from build123d import *

# Parameters (mm, degrees)
ESQUISSE1_W             = 10
ESQUISSE1_H             = 5
BOSS_EXTRU_1_DEPTH      = 8
ESQUISSE2_W             = 6.6
ESQUISSE2_H             = 0.8
ENL_V_MAT_EXTRU_1_DEPTH = 8
ENL_V_MAT_EXTRU_2_DEPTH = 6.5
ESQUISSE5_W             = 6
ESQUISSE5_H             = 0.5
ENL_V_MAT_EXTRU_3_DEPTH = 1
ESQUISSE6_W             = 5.6
ESQUISSE6_H             = 0.5
ENL_V_MAT_EXTRU_4_DEPTH = 3
ESQUISSE7_W             = 0.8
ESQUISSE7_H             = 1
ENL_V_MAT_EXTRU_5_DEPTH = 10
ESQUISSE8_W             = 6.8
ESQUISSE8_H             = 4.2
ENL_V_MAT_EXTRU_6_DEPTH = 1
BOSS_EXTRU_2_DEPTH      = 6.8
BOSS_EXTRU_3_DEPTH      = 2
BOSS_EXTRU_3_DEPTH_BACK = 2
ESQUISSE12_W            = 0.5
ESQUISSE12_H            = 4.2
BOSS_EXTRU_4_DEPTH      = 1
CHANFREIN1_SIZE         = 0.15
BOSS_EXTRU_5_DEPTH      = 0.5
BOSS_EXTRU_5_DEPTH_BACK = 6.3
ESQUISSE13_W            = 0.45
ESQUISSE13_H            = 0.45
ESQUISSE14_W            = 0.45
ESQUISSE14_H            = 0.43
BOSS_EXTRU_6_DEPTH      = 5.5
CONG_1_R                = 0.1
CHANFREIN2_SIZE         = 0.1


with BuildPart() as part:
    # Esquisse1 → Boss.-Extru.1 (new body)
    with BuildSketch(Plane(origin=(0, 0, 0), x_dir=(1, 0, 0), z_dir=(0, 1, 0))):
        with Locations((5, 2.5)):
            Rectangle(ESQUISSE1_W, ESQUISSE1_H)
    extrude(amount=BOSS_EXTRU_1_DEPTH)

    # Esquisse2 → Enlèv. mat.-Extru.1 (cut)
    with BuildSketch(Plane(origin=(0, 8, 0), x_dir=(1, 0, 0), z_dir=(0, 1, 0))):
        with Locations((5, 0.4)):
            Rectangle(ESQUISSE2_W, ESQUISSE2_H)
    extrude(amount=-ENL_V_MAT_EXTRU_1_DEPTH, mode=Mode.SUBTRACT)

    # Esquisse4 → Enlèv. mat.-Extru.2 (cut)
    with BuildSketch(Plane(origin=(0, 8, 0), x_dir=(1, 0, 0), z_dir=(0, 1, 0))):
        Polygon((0.5, 0.5), (1.2, 0.5), (1.2, 1.3), (8.8, 1.3), (8.8, 0.5), (9.5, 0.5), (9.5, 4.5), (0.5, 4.5), align=None)
    extrude(amount=-ENL_V_MAT_EXTRU_2_DEPTH, mode=Mode.SUBTRACT)

    # Esquisse5 → Enlèv. mat.-Extru.3 (cut)
    with BuildSketch(Plane(origin=(0, 8, 0), x_dir=(1, 0, 0), z_dir=(0, 1, 0))):
        with Locations((5, 4.75)):
            Rectangle(ESQUISSE5_W, ESQUISSE5_H)
    extrude(amount=-ENL_V_MAT_EXTRU_3_DEPTH, mode=Mode.SUBTRACT)

    # Esquisse6 → Enlèv. mat.-Extru.4 (cut)
    with BuildSketch(Plane(origin=(0, 8, 0), x_dir=(1, 0, 0), z_dir=(0, 1, 0))):
        with Locations((5, 1.05)):
            Rectangle(ESQUISSE6_W, ESQUISSE6_H)
    extrude(amount=-ENL_V_MAT_EXTRU_4_DEPTH, mode=Mode.SUBTRACT)

    # Esquisse7 → Enlèv. mat.-Extru.5 (cut)
    with BuildSketch(Plane(origin=(10, 0, 0), x_dir=(0, 0, -1), z_dir=(1, 0, 0))):
        with Locations((0.4, 0.5)):
            Rectangle(ESQUISSE7_W, ESQUISSE7_H)
    extrude(amount=-ENL_V_MAT_EXTRU_5_DEPTH, mode=Mode.SUBTRACT)

    # Esquisse8 → Enlèv. mat.-Extru.6 (cut)
    with BuildSketch(Plane.XZ):
        with Locations((5, -2.9)):
            Rectangle(ESQUISSE8_W, ESQUISSE8_H)
    extrude(amount=-ENL_V_MAT_EXTRU_6_DEPTH, mode=Mode.SUBTRACT)

    # Esquisse9 → Boss.-Extru.2 (add)
    with BuildSketch(Plane(origin=(1.6, 0, 0), x_dir=(0, 0, -1), z_dir=(1, 0, 0))):
        Polygon((4.7, 1), (3.9, 0.2), (1.9, 0.2), (1.1, 1), align=None)
    extrude(amount=BOSS_EXTRU_2_DEPTH)

    # Esquisse11 → Boss.-Extru.3 (add, two sides: drawn at the far end of the back side and taken through both)
    with BuildSketch(Plane(origin=(5, 0, 0), x_dir=(0, 0, -1), z_dir=(1, 0, 0)).offset(-BOSS_EXTRU_3_DEPTH_BACK)):
        Polygon((0.8, 5), (0.1, 3.4), (0.8, 3.4), align=None)
    extrude(amount=BOSS_EXTRU_3_DEPTH + BOSS_EXTRU_3_DEPTH_BACK)

    # Esquisse12 → Boss.-Extru.4 (add)
    with BuildSketch(Plane(origin=(0, 1, 0), x_dir=(1, 0, 0), z_dir=(0, 1, 0))):
        with Locations((5, 2.9)):
            Rectangle(ESQUISSE12_W, ESQUISSE12_H)
        with Locations((3.175, 2.9)):
            Rectangle(ESQUISSE12_W, ESQUISSE12_H)
        with Locations((6.825, 2.9)):
            Rectangle(ESQUISSE12_W, ESQUISSE12_H)
    extrude(amount=-BOSS_EXTRU_4_DEPTH)

    # Chanfrein1
    chanfrein1_edges = [part.edges().sort_by_distance(p)[0] for p in [
        (2.2, 8, -1.05),
        (7.8, 8, -1.05),
    ]]
    chamfer(chanfrein1_edges, length=CHANFREIN1_SIZE)

    # Esquisse13 → Boss.-Extru.5 (add, two sides: drawn at the far end of the back side and taken through both)
    with BuildSketch(Plane.XZ.offset(-0.2).offset(-BOSS_EXTRU_5_DEPTH_BACK)):
        with Locations((4, -2.9)):
            Rectangle(ESQUISSE13_W, ESQUISSE13_H)
        with Locations((2, -2.9)):
            Rectangle(ESQUISSE13_W, ESQUISSE13_H)
        with Locations((8, -2.9)):
            Rectangle(ESQUISSE13_W, ESQUISSE13_H)
        with Locations((6, -2.9)):
            Rectangle(ESQUISSE13_W, ESQUISSE13_H)
    extrude(amount=BOSS_EXTRU_5_DEPTH + BOSS_EXTRU_5_DEPTH_BACK)

    # Esquisse14 → Boss.-Extru.6 (add)
    with BuildSketch(Plane(origin=(0, 0, -3.125), x_dir=(-1, 0, 0), z_dir=(0, 0, -1))):
        with Locations((-8, -0.085)):
            Rectangle(ESQUISSE14_W, ESQUISSE14_H)
        with Locations((-6, -0.085)):
            Rectangle(ESQUISSE14_W, ESQUISSE14_H)
        with Locations((-4, -0.085)):
            Rectangle(ESQUISSE14_W, ESQUISSE14_H)
        with Locations((-2, -0.085)):
            Rectangle(ESQUISSE14_W, ESQUISSE14_H)
    extrude(amount=BOSS_EXTRU_6_DEPTH)

    # Congé1
    # the kernel refuses this fillet: 0.1 mm, written as the material it adds along each edge
    with BuildSketch(Plane(origin=(7.775, 0.13, -3.125), x_dir=(0, 1, 0), z_dir=(1, 0, 0)), Plane(origin=(5.775, 0.13, -3.125), x_dir=(0, 1, 0), z_dir=(1, 0, 0))) as cong_1_piece_1:
        with BuildLine():
            CenterArc((0.1, -0.09539392), CONG_1_R, 107.457603124, 72.542396876)
            Line((0, -0.09539392), (0, 0))
            Line((0, 0), (0.07, 0))
        make_face()
    extrude(amount=0.45)
    with BuildSketch(Plane(origin=(3.775, 0.13, -3.125), x_dir=(0, 0, -1), z_dir=(1, 0, 0)), Plane(origin=(1.775, 0.13, -3.125), x_dir=(0, 0, -1), z_dir=(1, 0, 0))) as cong_1_piece_2:
        with BuildLine():
            CenterArc((0.09539392, 0.1), CONG_1_R, 197.457603124, 72.542396876)
            Line((0, 0.07), (0, 0))
            Line((0, 0), (0.09539392, 0))
        make_face()
    extrude(amount=0.45)
    # the kernel refuses this fillet: 0.1 mm, written as the material it takes off along each edge
    with BuildSketch(Plane(origin=(3.525, -0.3, -2.675), x_dir=(0, 1, 0), z_dir=(1, 0, 0)), Plane(origin=(1.525, -0.3, -2.675), x_dir=(0, 1, 0), z_dir=(1, 0, 0))) as cong_1_2_piece_1:
        with BuildLine():
            CenterArc((CONG_1_R, -CONG_1_R), CONG_1_R, 90, 90)
            Line((0, -CONG_1_R), (0, 0))
            Line((0, 0), (CONG_1_R, 0))
        make_face()
    extrude(amount=0.95, mode=Mode.SUBTRACT)
    with BuildSketch(Plane(origin=(8.475, -0.3, -2.675), x_dir=(0, 1, 0), z_dir=(-1, 0, 0)), Plane(origin=(6.475, -0.3, -2.675), x_dir=(0, 1, 0), z_dir=(-1, 0, 0))) as cong_1_2_piece_2:
        with BuildLine():
            CenterArc((CONG_1_R, CONG_1_R), CONG_1_R, 180, 90)
            Line((0, CONG_1_R), (0, 0))
            Line((0, 0), (CONG_1_R, 0))
        make_face()
    extrude(amount=0.95, mode=Mode.SUBTRACT)

    # Chanfrein2
    chanfrein2_edges = [part.edges().sort_by_distance(p)[0] for p in [
        (4.225, 6.5, -2.9),
        (4, 6.5, -3.125),
        (3.775, 6.5, -2.9),
        (4, 6.5, -2.675),
        (2.225, 6.5, -2.9),
        (2, 6.5, -3.125),
        (1.775, 6.5, -2.9),
        (2, 6.5, -2.675),
        (7.775, 6.5, -2.9),
        (8, 6.5, -2.675),
        (8.225, 6.5, -2.9),
        (8, 6.5, -3.125),
        (5.775, 6.5, -2.9),
        (6, 6.5, -2.675),
        (6.225, 6.5, -2.9),
        (6, 6.5, -3.125),
        (8.225, -0.085, -8.625),
        (8, -0.3, -8.625),
        (7.775, -0.085, -8.625),
        (8, 0.13, -8.625),
        (6.225, -0.085, -8.625),
        (6, -0.3, -8.625),
        (5.775, -0.085, -8.625),
        (6, 0.13, -8.625),
        (4.225, -0.085, -8.625),
        (4, -0.3, -8.625),
        (3.775, -0.085, -8.625),
        (4, 0.13, -8.625),
        (2.225, -0.085, -8.625),
        (2, -0.3, -8.625),
        (1.775, -0.085, -8.625),
        (2, 0.13, -8.625),
    ]]
    chamfer(chanfrein2_edges, length=CHANFREIN2_SIZE)


solid = part.part
Check sheet for the modelled part. Datum: model origin and axes. Units: mm. A direction names the side the tool comes from. Round coordinates to 2 decimals unless told otherwise and drop trailing zeros. Order: outer loops, then holes, each group sorted by start corner. A loop starts at its lowest first (then second) coordinate and runs counter-clockwise, first axis right, second up.
Q1. Cross-section at C-C, the plane z = -5.25. Enter the section's corners in (x, y) (3 decimals), plus the area to 3 significant figures.
Filled sheet:
outline: (1.775, -0.3) - (2.225, -0.3) - (2.225, 0.13) - (1.775, 0.13) - close; (3.775, -0.3) - (4.225, -0.3) - (4.225, 0.13) - (3.775, 0.13) - close; (5.775, -0.3) - (6.225, -0.3) - (6.225, 0.13) - (5.775, 0.13) - close; (7.775, -0.3) - (8.225, -0.3) - (8.225, 0.13) - (7.775, 0.13) - close
area: 0.774 mm2
Q2. Cross-section at D-D, the plane x = 5.5. Enter the section's corners in (y, z), plus the area to 3 significant figures.
Filled sheet:
outline: (0.2, -3.9) - (1, -4.7) - (1, -5) - (7, -5) - (7, -4.5) - (1.5, -4.5) - (1.5, -1.3) - (5, -1.3) - (5, -0.8) - (3.4, -0.1) - (3.4, -0.8) - (1, -0.8) - (1, -1.1) - (0.2, -1.9) - close
area: 9.40 mm2
Q3. Scan lines: L1, parallel to X at y = 6, z = -0.75; L2, parallel to Z at x = 0.75, y = 5.5; L3, parallel to X at y = 3.75, z = -1.5. Record each from-to range of solid material in increasing order.
Filled sheet:
L1: x = 0 to 0.5, 1.2 to 1.7, 8.3 to 8.8, 9.5 to 10
L2: z = -5 to -4.5, -0.5 to 0
L3: x = 0 to 0.5, 9.5 to 10
Q4. Depth check by flat-ended pin: P1, Ø0.6, axis at y = 3.5, z = -0.5, coming from the -X side; P2, Ø0.5, axis at x = 0.5, z = -2, coming from the -Y side. Enter the tip coordinate at first touch or a pass-through.
Filled sheet:
P1: stops at x = 0
P2: stops at y = 0
Q5. Set-up check for faces 1 (the face through (9.5, 5, -2)), 2 (the face through (4.4, 0.2, -2.9)), 3 (the face through (7.7, 0.6, -1.5)), 4 (the face through (0.8, 0.5, -0.8)): record each of +Z, -Z, +X, -X, +Y, -Y from which the full face is reachable in a straight line by a thin tool's end or side.
Filled sheet:
face 1: +Y
face 2: none
face 3: +Z, -Y
face 4: +Z, +X, -X, -Y
Q6. Draft check along X on faces 5 (the face through (1, 0, -3)), 6 (the face through (5, 5, -4.5)), 7 (the face through (7.6, 0.2, -2.9)). Enter one of: pulls with the +X half, pulls with the -X half, needs draft (parallel to the pull), parting line crosses it, or undercut.
Filled sheet:
face 5: needs draft
face 6: undercut
face 7: undercut
Q7. Cross-section at A-A, the plane y = 2.5. Give the number of separate pieces and of enclosed holes in the cut face, plus the area to 3 significant figures.
Filled sheet:
separate pieces: 5
enclosed holes: 1
area: 15.6 mm2
Q8. Cross-section at B-B, the plane y = 7.25. Enter the section's corners in (x, z), plus the area to 3 significant figures.
Filled sheet:
outline: (0, -5) - (2, -5) - (2, -4.5) - (0.5, -4.5) - (0.5, -0.5) - (1.2, -0.5) - (1.2, -1.3) - (2.2, -1.3) - (2.2, -0.8) - (1.7, -0.8) - (1.7, 0) - (0, 0) - close; (7.8, -1.3) - (8.8, -1.3) - (8.8, -0.5) - (9.5, -0.5) - (9.5, -4.5) - (8, -4.5) - (8, -5) - (10, -5) - (10, 0) - (8.3, 0) - (8.3, -0.8) - (7.8, -0.8) - close
area: 9.00 mm2
